Geometry check sheet. Reference: the model listing, model coordinates, mm. Face numbers are marked on the shaded views. A direction names the side the tool comes from. Round coordinates to 2 decimals unless told otherwise and drop trailing zeros. Write each loop counter-clockwise with the first axis right and the second up, starting at its lowest first coordinate (ties: lowest second). Pieces come first, ordered by that corner, then holes. Notation, with made-up numbers: M 45,1 L 71,1 A8 cw 71,11 Z; hole C 78.5,18.5 d9. An arc over 180 degrees is marked long. Answer in a Markdown table with one row per item. Add a question column.
from build123d import *

# Parameters (mm, degrees)
SKETCH_R     = 2.2
PAD_DEPTH    = 3.5
SKETCH001_W  = 15
SKETCH001_H  = 6.5
SKETCH001_R  = 1.55
PAD001_DEPTH = 5
SKETCH002_W  = 5.5
SKETCH002_H  = 5.5
POCKET_DEPTH = 2
PAD002_DEPTH = 3


with BuildPart() as part:
    # Sketch → Pad (new body)
    with BuildSketch(Plane.XZ):
        with BuildLine():
            Line((10.6, -8.5), (10.6, -15))
            Line((10.6, -15), (15.6, -15))
            Line((15.6, -15), (15.6, 0))
            Line((5.5, 0), (15.6, 0))
            ThreePointArc((3.1, 2.4), (3.802944, 0.702944), (5.5, 0))
            Line((3.1, 5.5), (3.1, 2.4))
            Line((-3.1, 5.5), (3.1, 5.5))
            Line((-3.1, -2.4), (-3.1, 5.5))
            ThreePointArc((-3.1, -2.4), (-2.192031, -4.592031), (0, -5.5))
            Line((7.6, -5.5), (0, -5.5))
            ThreePointArc((10.6, -8.5), (9.72132, -6.37868), (7.6, -5.5))
        make_face()
        with Locations((0, 2.4)):
            Circle(SKETCH_R, mode=Mode.SUBTRACT)
        with Locations((0, -2.4)):
            Circle(SKETCH_R, mode=Mode.SUBTRACT)
    extrude(amount=PAD_DEPTH)

    # Sketch001 (on Face4 of Pad) → Pad001 (join)
    with BuildSketch(Plane(origin=(15.6, 0, 0), x_dir=(0, 0, 1), z_dir=(1, 0, 0))):
        with Locations((-7.5, 6.75)):
            Rectangle(SKETCH001_W, SKETCH001_H)
        with Locations((-4, 6.75)):
            Circle(SKETCH001_R, mode=Mode.SUBTRACT)
        with Locations((-11, 6.75)):
            Circle(SKETCH001_R, mode=Mode.SUBTRACT)
    extrude(amount=-PAD001_DEPTH)

    # Sketch002 (on Face12 of Pad001) → Pocket (cut)
    with BuildSketch(Plane(origin=(10.6, 0, 0), x_dir=(0, 0, -1), z_dir=(-1, 0, 0))):
        with Locations((4, 6.75)):
            Rectangle(SKETCH002_W, SKETCH002_H)
        with Locations((11, 6.75)):
            Rectangle(SKETCH002_W, SKETCH002_H)
    extrude(amount=-POCKET_DEPTH, mode=Mode.SUBTRACT)

    # Sketch003 (on Face5 of Pocket) → Pad002 (join)
    with BuildSketch(Plane.XZ.offset(3.5)):
        with BuildLine():
            Line((-3.1, 5.5), (3.1, 5.5))
            Line((3.1, 5.5), (3.1, -5.5))
            Line((3.1, -5.5), (0, -5.5))
            ThreePointArc((-3.1, -2.4), (-2.192031, -4.592031), (0, -5.5))
            Line((-3.1, -2.4), (-3.1, 5.5))
        make_face()
    extrude(amount=PAD002_DEPTH)


solid = part.part
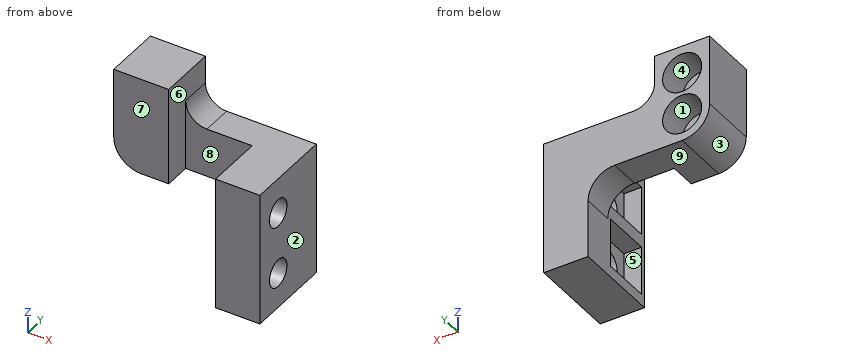
Item 1: Section check D-D, the plane y = -2. Record the boundary of the cut face in (x, z).
Item 2: Section check B-B, the plane z = -11. Record the boundary of the cut face in (x, y), and give its area (3 significant figures).
Item 3: Gauge pin test, flat ends, axial feed: pin 1 Ø1.9 at (x, z) = (1, -0.5) entering from -Y; pin 2 Ø2 at (y, z) = (-2, -6) entering from -X; pin 3 Ø5 at (x, y) = (11, -4) entering from +Z; pin 4 Ø1.5 at (x, y) = (9, -7) entering from -Z. Record the tip position at first contact, or that the pin passes through.
Item 4: Mould release check, pull along X, two halves, no side actions. Record for the marked faces 1, 2, 3 and 4: +X half, -X half, draft (parallel to the pull), parting line (faces both ways), or undercut.
Item 5: Access from +Z, -Z, +X, -X, +Y, -Y to the whole of each face (thin tool, end or side, straight path). Record for the marked faces 5, 6, 7, 8 and 9.
Item 6: Section check A-A, the plane y = -6.75. Record the boundary of the cut face in (x, z).
Item 7: Scan lines: probe 1 along Z at (x, y) = (14.3, -6.75); probe 2 along Z at (x, y) = (0, -0.9); probe 3 along Y at (x, z) = (14.3, -11). Record each from-to range of solid material in increasing order. Write a range as from..to.
Item 8: Section check C-C, the plane x = 11.5. Record the boundary of the cut face in (y, z).
Result sheet:
| question | item | result |
|---|---|---|
| 1 | outline | M -3.1,-2.4 A3.1 ccw 0,-5.5 L 7.6,-5.5 A3 cw 10.6,-8.5 L 10.6,-15 L 15.6,-15 L 15.6,0 L 5.5,0 A2.4 cw 3.1,2.4 L 3.1,5.5 L -3.1,5.5 Z; hole C 0,-2.4 d4.4; hole C 0,2.4 d4.4 |
| 2 | outline | M 10.6,-10 L 15.6,-10 L 15.6,-8.3 L 12.6,-8.3 L 12.6,-9.5 L 10.6,-9.5 Z; M 10.6,-4 L 12.6,-4 L 12.6,-5.2 L 15.6,-5.2 L 15.6,0 L 10.6,0 Z |
| 2 | area | 29.7 mm^2 |
| 3 | pin 1 | stops at y = -6.5 |
| 3 | pin 2 | stops at x = -1.69 |
| 3 | pin 3 | stops at z = 0 |
| 3 | pin 4 | passes through |
| 4 | face 1 | undercut |
| 4 | face 2 | +X half |
| 4 | face 3 | -X half |
| 4 | face 4 | undercut |
| 5 | face 5 | -X |
| 5 | face 6 | +Z, -Y |
| 5 | face 7 | +Z, -Z, -X, -Y |
| 5 | face 8 | +Z, -Z, -Y |
| 5 | face 9 | -Z, -X, +Y, -Y |
| 6 | outline | M 10.6,-15 L 15.6,-15 L 15.6,-12.55 L 12.6,-12.55 L 12.6,-13.75 L 10.6,-13.75 Z; M 10.6,-8.25 L 12.6,-8.25 L 12.6,-9.45 L 15.6,-9.45 L 15.6,-5.55 L 12.6,-5.55 L 12.6,-6.75 L 10.6,-6.75 Z; M 10.6,-1.25 L 12.6,-1.25 L 12.6,-2.45 L 15.6,-2.45 L 15.6,0 L 10.6,0 Z |
| 7 | probe 1 | z = -15..-12.55, -9.45..-5.55, -2.45..0 |
| 7 | probe 2 | z = -5.5..-4.6, -0.2..0.2, 4.6..5.5 |
| 7 | probe 3 | y = -10..-8.3, -5.2..0 |
| 8 | outline | M -10,-15 L 0,-15 L 0,0 L -10,0 Z; hole M -9.5,-13.75 L -4,-13.75 L -4,-8.25 L -9.5,-8.25 Z; hole M -9.5,-6.75 L -4,-6.75 L -4,-1.25 L -9.5,-1.25 Z |
